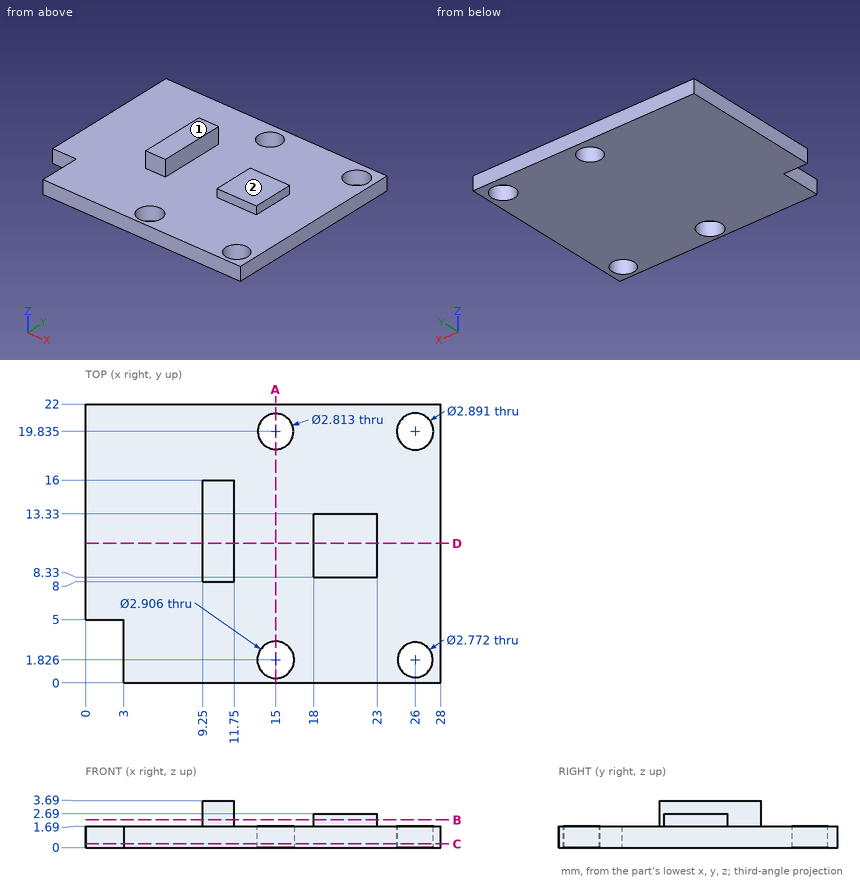
The figure shows three views and two pictorial views of one solid part (mm, origin at its lowest corner). Answer the questions. A direction names the side the tool comes from. Coordinates: 2 decimals unless noted, no trailing zeros. Loops run counter-clockwise (first coordinate to the right, second up) from the corner with the lowest first, then second, coordinate; pieces in that order, holes last. Notation, with made-up numbers: M 39,-29.5 L 44,-29.5 A18 ccw 44,-8.5 Z; hole C 39,69.25 d2. An arc over 180 degrees is marked long. Use CSV: the item, a comma, the result in double quotes. Start each with the question number.
(1) Consider line 1 (Y direction, x = 15, z = 0.75); line 2 (Y direction, x = 26, z = 1.25); line 3 (X direction, y = 11.5, z = 1.95). Determine where each line is inside the solid, lowest interval first.
(2) Find section B-B, the plane z = 2.2. Give the vertices of the cut face in (x, y), then the cut area to 3 significant figures.
(3) Find section D-D, the plane y = 11. Give the vertices of the cut face in (x, z).
(4) Find section A-A, the plane x = 15. Give the vertices of the cut face in (y, z).
(5) Given pin 1 Ø0.8 at (y, z) = (11.5, 2.5) entering from -X; pin 2 Ø1 at (x, y) = (5.5, 13) entering from -Z; pin 3 Ø1.5 at (x, y) = (20, 12) entering from +Z; pin 4 Ø1.9 at (y, z) = (3, 0.5) entering from -X, each flat-ended and moving along its own axis, determine where each tip first touches the part or whether it passes through.
(6) For the marked faces 1 and 2, determine the directions among +Z, -Z, +X, -X, +Y, -Y from which every point of the face is accessible in a straight line to the end or side of a thin tool.
(7) Find section C-C, the plane z = 0.3. Give the vertices of the cut face in (x, y) (1 decimal).
Recorded:
1,line 1,"y = 0 to 0.37, 3.28 to 18.43, 21.24 to 22"
1,line 2,"y = 0 to 0.44, 3.21 to 18.39, 21.28 to 22"
1,line 3,"x = 9.25 to 11.75, 18 to 23"
2,outline,"M 9.25,8 L 11.75,8 L 11.75,16 L 9.25,16 Z; M 18,8.33 L 23,8.33 L 23,13.33 L 18,13.33 Z"
2,area,"45.0 mm^2"
3,outline,"M 0,0 L 28,0 L 28,1.69 L 23,1.69 L 23,2.69 L 18,2.69 L 18,1.69 L 11.75,1.69 L 11.75,3.69 L 9.25,3.69 L 9.25,1.69 L 0,1.69 Z"
4,outline,"M 0,0 L 0.37,0 L 0.37,1.69 L 0,1.69 Z; M 3.28,0 L 18.43,0 L 18.43,1.69 L 3.28,1.69 Z; M 21.24,0 L 22,0 L 22,1.69 L 21.24,1.69 Z"
5,pin 1,"stops at x = 9.25"
5,pin 2,"stops at z = 0"
5,pin 3,"stops at z = 2.69"
5,pin 4,"stops at x = 3"
6,face 1,"+Z, +X, -X, +Y, -Y"
6,face 2,"+Z, +X, +Y, -Y"
7,outline,"M 0,5 L 3,5 L 3,0 L 28,0 L 28,22 L 0,22 Z; hole C 15,1.8 d2.9; hole C 15,19.8 d2.8; hole C 26,1.8 d2.8; hole C 26,19.8 d2.9"
